Study the drawing (mm; zero at the part's minimum x, y, z) and answer. Give positions to 0.01 mm unless a question says otherwise; leave off trailing zeros. Order: outer loops, then holes, each group sorted by start corner. A loop starts at its lowest first (then second) coordinate and runs counter-clockwise, first axis right, second up. Notation, with made-up numbers: (58, 40.5) -> (95, 40.5) arc R23 ccw to (95, 50.5) -> close; hole circle Ø7 at (28.5, 44). An arc over 180 degrees is marked (long way). Use a Markdown table: item, result. Add a question column.
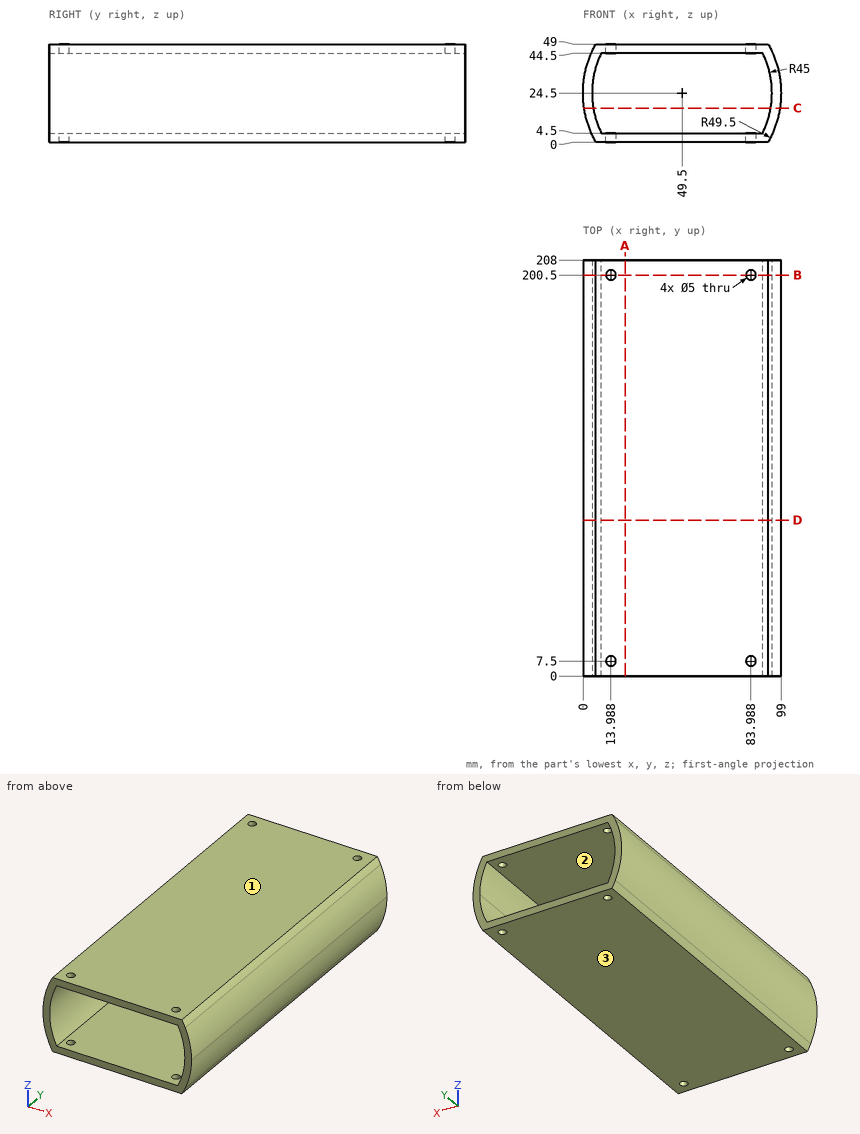
1) The part is cut by section A-A, the plane x = 21. Determine the outline of the cut face in (y, z).
2) The part is cut by section B-B, the plane y = 200.5. Determine the outline of the cut face in (x, z), then the cut area to 3 significant figures.
3) Flat-ended cylindrical pins translate along their axes: pin 1 (3 mm diameter, centred on x = 13.99, y = 7.5, fed in from -Z); pin 2 (3 mm diameter, centred on y = 184, z = 39, fed in from -X); pin 3 (8 mm diameter, centred on y = 87.5, z = 29, fed in from +X); pin 4 (10 mm diameter, centred on y = 40, z = 6, fed in from -X). Find the tip coordinate at first contact, or state that the pin passes through.
4) The part is cut by section C-C, the plane z = 17. Determine the outline of the cut face in (x, y), then the cut area to 3 significant figures.
5) Determine the mould class of the marked faces 1, 2 and 3 for opening direction Z: released by +Z, released by -Z, zero draft, split by the parting line, or undercut.
6) Straight lines are drawn through the part: line 1 (Z direction, x = 17.5, y = 45); line 2 (X direction, y = 7, z = 47); line 3 (X direction, y = 130, z = 26) (1 decimal). For each, find the intervals that lie inside material, in ascending order.
7) The part is cut by section D-D, the plane y = 78. Determine the outline of the cut face in (x, z), then the cut area to 3 significant figures.
A:
| question | item | result |
|---|---|---|
| 1 | outline | (0, 0) -> (208, 0) -> (208, 4.5) -> (0, 4.5) -> close; (0, 44.5) -> (208, 44.5) -> (208, 49) -> (0, 49) -> close |
| 2 | outline | (6.49, 0) -> (11.49, 0) -> (11.49, 4.5) -> (9.19, 4.5) arc R45 cw to (9.19, 44.5) -> (11.49, 44.5) -> (11.49, 49) -> (6.49, 49) arc R49.5 ccw to start; (16.49, 0) -> (81.49, 0) -> (81.49, 4.5) -> (16.49, 4.5) -> close; (16.49, 44.5) -> (81.49, 44.5) -> (81.49, 49) -> (16.49, 49) -> close; (86.49, 0) -> (92.51, 0) arc R49.5 ccw to (92.51, 49) -> (86.49, 49) -> (86.49, 44.5) -> (89.81, 44.5) arc R45 cw to (89.81, 4.5) -> (86.49, 4.5) -> close |
| 2 | area | 1,080 mm^2 |
| 3 | pin 1 | through |
| 3 | pin 2 | x = 1.74 |
| 3 | pin 3 | x = 99 |
| 3 | pin 4 | x = 1.88 |
| 4 | outline | (0.57, 0) -> (5.13, 0) -> (5.13, 208) -> (0.57, 208) -> close; (93.87, 0) -> (98.43, 0) -> (98.43, 208) -> (93.87, 208) -> close |
| 4 | area | 1,900 mm^2 |
| 5 | face 1 | released by +Z |
| 5 | face 2 | undercut |
| 5 | face 3 | released by -Z |
| 6 | line 1 | 0 to 4.5, 44.5 to 49 |
| 6 | line 2 | 5.41 to 11.54, 16.44 to 81.54, 86.44 to 93.59 |
| 6 | line 3 | 0 to 4.5, 94.5 to 99 |
| 7 | outline | (6.49, 0) -> (92.51, 0) arc R49.5 ccw to (92.51, 49) -> (6.49, 49) arc R49.5 ccw to start; hole (9.19, 4.5) -> (89.81, 4.5) arc R45 ccw to (89.81, 44.5) -> (9.19, 44.5) arc R45 ccw to start |
| 7 | area | 1,170 mm^2 |
